The listing builds one solid part. Answer for the finished solid, in the listing's coordinates (mm). Face numbers are marked on the shaded views. A direction names the side the tool comes from. Give positions to 0.01 mm unless a question says otherwise; leave off trailing zeros. Loops run counter-clockwise (first coordinate to the right, second up) from the corner with the lowest first, then second, coordinate; pieces in that order, holes last. Notation, with made-up numbers: (-25, 74.5) - (-10, 74.5) arc R26 cw to (-10, 94.5) - close; hole circle Ø3 at (85, -0.5). An arc over 180 degrees is marked (long way). One line per item, written item: value. Start each with the question number.
from build123d import *

# Parameters (mm, degrees)
SCHIZZO1_R                   = 1.5
ESTRUSIONE_ESTRUSIONE1_DEPTH = 0.6
SCHIZZO2_R                   = 5
ESTRUSIONE_ESTRUSIONE2_DEPTH = 0.6
SCHIZZO3_R                   = 5
SCHIZZO3_R_2                 = 4.8
ESTRUSIONE_ESTRUSIONE3_DEPTH = 10.8


with BuildPart() as part:
    # Schizzo1 → Estrusione-Estrusione1 (new body)
    # profile 1 of 5: a face of its own
    with BuildSketch(Plane(origin=(0, 0, 0), x_dir=(1, 0, 0), z_dir=(0, 1, 0))):
        with BuildLine():
            ThreePointArc((2.561737691, 2), (-3.25, 0), (2.561737691, -2))
            Line((2.561737691, -2), (2.561737691, 2))
        make_face()
        with Locations(Location((0, 0, 0), (0, 0, 270))):
            Circle(SCHIZZO1_R, mode=Mode.SUBTRACT)
    # profile 2 of 5: a face of its own
    with BuildSketch(Plane(origin=(0, 0, 0), x_dir=(1, 0, 0), z_dir=(0, 1, 0))):
        with BuildLine():
            ThreePointArc((3.25, 0), (3.073121174, -1.057556737), (2.561737691, -2))
            Line((2.561737691, -2), (24.938262309, -2))
            ThreePointArc((24.938262309, -2), (24.25, 0), (24.938262309, 2))
            Line((24.938262309, 2), (2.561737691, 2))
            ThreePointArc((2.561737691, 2), (3.073121174, 1.057556737), (3.25, 0))
        make_face()
    # profile 3 of 5: a face of its own
    with BuildSketch(Plane(origin=(0, 0, 0), x_dir=(1, 0, 0), z_dir=(0, 1, 0))):
        with BuildLine():
            Line((2.561737691, 2), (2.561737691, -2))
            ThreePointArc((2.561737691, -2), (3.073121174, -1.057556737), (3.25, 0))
            ThreePointArc((3.25, 0), (3.073121174, 1.057556737), (2.561737691, 2))
        make_face()
    # profile 4 of 5: a face of its own
    with BuildSketch(Plane(origin=(0, 0, 0), x_dir=(1, 0, 0), z_dir=(0, 1, 0))):
        with BuildLine():
            Line((24.938262309, 2), (24.938262309, -2))
            ThreePointArc((24.938262309, -2), (28.557556737, -3.073121174), (30.75, 0))
            ThreePointArc((30.75, 0), (28.557556737, 3.073121174), (24.938262309, 2))
        make_face()
        with Locations(Location((27.5, 0, 0), (0, 0, 270))):
            Circle(SCHIZZO1_R, mode=Mode.SUBTRACT)
    # profile 5 of 5: a face of its own
    with BuildSketch(Plane(origin=(0, 0, 0), x_dir=(1, 0, 0), z_dir=(0, 1, 0))):
        with BuildLine():
            ThreePointArc((24.938262309, 2), (24.25, 0), (24.938262309, -2))
            Line((24.938262309, -2), (24.938262309, 2))
        make_face()
    extrude(amount=ESTRUSIONE_ESTRUSIONE1_DEPTH)

    # Schizzo2 → Estrusione-Estrusione2 (add)
    with BuildSketch(Plane(origin=(0, 0.6, 0), x_dir=(1, 0, 0), z_dir=(0, 1, 0))):
        with Locations(Location((13.75, 0, 0), (0, 0, 23.578178478))):
            Circle(SCHIZZO2_R)
    extrude(amount=ESTRUSIONE_ESTRUSIONE2_DEPTH)

    # Schizzo3 → Estrusione-Estrusione3 (add)
    with BuildSketch(Plane(origin=(0, 1.2, 0), x_dir=(1, 0, 0), z_dir=(0, 1, 0))):
        with Locations(Location((13.75, 0, 0), (0, 0, 23.578178478))):
            Circle(SCHIZZO3_R)
        with Locations(Location((13.75, 0, 0), (0, 0, 90))):
            Circle(SCHIZZO3_R_2, mode=Mode.SUBTRACT)
    extrude(amount=ESTRUSIONE_ESTRUSIONE3_DEPTH)


solid = part.part
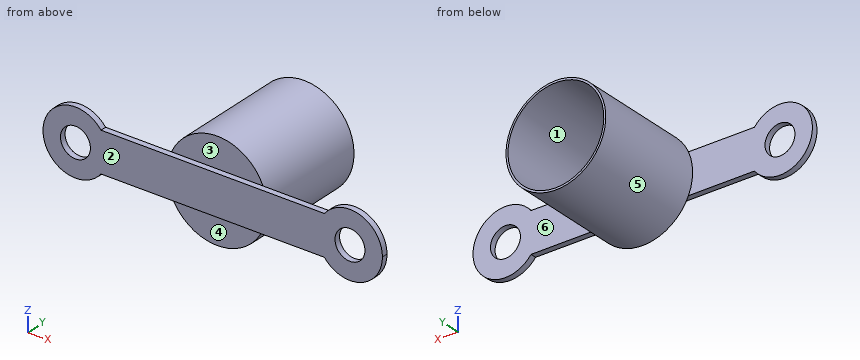
1. A cutting plane is placed at B-B (z = -2.5). Determine the outline of the cut face in (x, y).
2. A cutting plane is placed at D-D (x = 13.75). Determine the outline of the cut face in (y, z).
3. A cutting plane is placed at A-A (x = 27.5). Determine the outline of the cut face in (y, z).
4. For the marked faces 1, 2 and 3, determine the directions among +Z, -Z, +X, -X, +Y, -Y from which every point of the face is accessible in a straight line to the end or side of a thin tool.
5. A cutting plane is placed at C-C (y = 6.25). Determine the outline of the cut face in (x, z), plus the area to 3 significant figures.
6. Determine the mould class of the marked faces 4, 5 and 6 for opening direction X: released by +X, released by -X, zero draft, split by the parting line, or undercut.
7. Find the intervals of material crossed by L1, parallel to Y at x = 17, z = 3.25; L2, parallel to Z at x = 16, y = 4; L3, parallel to Y at x = 8.5, z = -0.5, in increasing order. Write a range as [from, to].
8. Flat-ended cylindrical pins translate along their axes: pin 1 (2 mm diameter, centred on x = 9.5, y = 5.5, fed in from +Z); pin 2 (1.9 mm diameter, centred on x = 5, z = -1.5, fed in from +Y); pin 3 (3 mm diameter, centred on x = 8.5, y = 4.5, fed in from +Z); pin 4 (2.5 mm diameter, centred on x = 0, z = 0, fed in from +Y). Find the tip coordinate at first contact, or state that the pin passes through.
Results below:
1. outline: (-2.08, 0) - (2.08, 0) - (2.08, 0.6) - (-2.08, 0.6) - close; (9.42, 0.6) - (18.08, 0.6) - (18.08, 12) - (17.85, 12) - (17.85, 1.2) - (9.65, 1.2) - (9.65, 12) - (9.42, 12) - close; (25.42, 0) - (29.58, 0) - (29.58, 0.6) - (25.42, 0.6) - close
2. outline: (0, -2) - (0.6, -2) - (0.6, -5) - (12, -5) - (12, -4.8) - (1.2, -4.8) - (1.2, 4.8) - (12, 4.8) - (12, 5) - (0.6, 5) - (0.6, 2) - (0, 2) - close
3. outline: (0, -3.25) - (0.6, -3.25) - (0.6, -1.5) - (0, -1.5) - close; (0, 1.5) - (0.6, 1.5) - (0.6, 3.25) - (0, 3.25) - close
4. face 1: +Y
4. face 2: +Z, -Z, +X, -X, -Y
4. face 3: +Z, -Y
5. outline: circle Ø10 at (13.75, 0); hole circle Ø9.6 at (13.75, 0)
5. area: 6.16 mm^2
6. face 4: undercut
6. face 5: split by the parting line
6. face 6: zero draft
7. L1: y = [0.6, 1.2]
7. L2: z = [-4.47, -4.24], [4.24, 4.47]
7. L3: y = [0, 0.6]
8. pin 1: stops at z = 3.8
8. pin 2: stops at y = 0.6
8. pin 3: stops at z = 3.31
8. pin 4: passes through
